from build123d import *

# Parameters (mm, degrees)
ESQUISSE1_W             = 27
ESQUISSE1_H             = 34
ESQUISSE1_R             = 10.5
BOSS_EXTRU_1_DEPTH      = 4
ESQUISSE2_W             = 27
ESQUISSE2_H             = 4
BOSS_EXTRU_2_DEPTH      = 8
BOSS_EXTRU_3_DEPTH      = 2
BOSS_EXTRU_4_DEPTH      = 2
CONG_1_R                = 10
ENL_V_MAT_EXTRU_1_DEPTH = 35.058772732


with BuildPart() as part:
    # Esquisse1 → Boss.-Extru.1 (new body)
    with BuildSketch(Plane(origin=(0, 0, 0), x_dir=(1, 0, 0), z_dir=(0, 1, 0))):
        with Locations((0.5, 3)):
            Rectangle(ESQUISSE1_W, ESQUISSE1_H)
        with Locations(Location((0, 0, 0), (0, 0, 270))):
            Circle(ESQUISSE1_R, mode=Mode.SUBTRACT)
    extrude(amount=BOSS_EXTRU_1_DEPTH)

    # Esquisse2 → Boss.-Extru.2 (add)
    with BuildSketch(Plane.XZ):
        with Locations((0.5, -18)):
            Rectangle(ESQUISSE2_W, ESQUISSE2_H)
    extrude(amount=BOSS_EXTRU_2_DEPTH)

    # Esquisse5 → Boss.-Extru.3 (add)
    with BuildSketch(Plane.ZY.offset(13)):
        Polygon((-16, 0), (-16, -5), (-11, 0), align=None)
    extrude(amount=-BOSS_EXTRU_3_DEPTH)

    # Esquisse6 → Boss.-Extru.4 (add)
    with BuildSketch(Plane(origin=(14, 0, 0), x_dir=(0, 0, -1), z_dir=(1, 0, 0))):
        Polygon((16, 0), (11, 0), (16, -5), align=None)
    extrude(amount=-BOSS_EXTRU_4_DEPTH)

    # Congé1
    cong_1_edges = [part.edges().sort_by_distance(p)[0] for p in [
        (-13, 2, 14),
        (14, 2, 14),
    ]]
    fillet(cong_1_edges, radius=CONG_1_R)

    # Esquisse7 → Enlèv. mat.-Extru.1 (cut, through all)
    with BuildSketch(Plane.XY.offset(-16)):
        with BuildLine():
            Line((-8, -2), (9, -2))
            ThreePointArc((9, -2), (11, -4), (9, -6))
            Line((9, -6), (-8, -6))
            ThreePointArc((-8, -6), (-10, -4), (-8, -2))
        make_face()
    extrude(amount=-ENL_V_MAT_EXTRU_1_DEPTH, mode=Mode.SUBTRACT)


solid = part.part
Here's how the part is built. I have some questions about the finished solid (model axes, mm). A direction names the side the tool comes from. Round coordinates to 2 decimals unless told otherwise and drop trailing zeros. Loops run counter-clockwise (first coordinate to the right, second up) from the corner with the lowest first, then second, coordinate; pieces in that order, holes last.
1. If we section it at B-B on y = -4: Write out the boundary of the cut face in (x, z).
Answer list:
outline: (-13, -20) - (-10, -20) - (-10, -16) - (-11, -16) - (-11, -15) - (-13, -15) - close; (11, -20) - (14, -20) - (14, -15) - (12, -15) - (12, -16) - (11, -16) - close
2. If we section it at A-A on z = 0: Write out the boundary of the cut face in (x, y).
Answer list:
outline: (-13, 0) - (-10.5, 0) - (-10.5, 4) - (-13, 4) - close; (10.5, 0) - (14, 0) - (14, 4) - (10.5, 4) - close
3. We'd pull the mould along Y, two halves only. Please class faces 1 (the face through (0, -2, -18)), 2 (the face through (-13, 1, -11)), 3 (the face through (0, 4, -11)): +Y half, -Y half, draft (parallel to the pull), parting line (faces both ways), or undercut.
Answer list:
face 1: undercut
face 2: draft
face 3: +Y half
4. If I drill on line 1 along Y through (x, z) = (-7, -17.5); line 2 along X through (y, z) = (2.95, 0); line 3 along X through (y, z) = (0.75, 9.5), over which ranges is the centre line in solid material (lowest first)?
Answer list:
line 1: y = -8 to -6, -2 to 4
line 2: x = -13 to -10.5, 10.5 to 14
line 3: x = -11.35 to -4.47, 4.47 to 12.35
5. Which directions (+Z, -Z, +X, -X, +Y, -Y) give clear straight access to the entire face, cutting with the end or side of a thin tool? Please do faces 4 (the face through (0, 2, 14)), 5 (the face through (0, -7, -16)), 6 (the face through (-10, -4, -18)).
Answer list:
face 4: +Z, +X, -X, +Y, -Y
face 5: +Z, -Y
face 6: +Z, -Z
6. If we section it at C-C on x = -7.25: Write out the boundary of the cut face in (y, z), plus the area to 3 significant figures.
Answer list:
outline: (-8, -20) - (-6, -20) - (-6, -16) - (-8, -16) - close; (-2, -20) - (4, -20) - (4, -7.6) - (0, -7.6) - (0, -16) - (-2, -16) - close; (0, 7.6) - (4, 7.6) - (4, 13.05) - (0, 13.05) - close
area: 87.4 mm2
7. If we section it at D-D on z = -8.5: Write out the boundary of the cut face in (x, y).
Answer list:
outline: (-13, 0) - (-6.16, 0) - (-6.16, 4) - (-13, 4) - close; (6.16, 0) - (14, 0) - (14, 4) - (6.16, 4) - close
8. For P1, Ø4, axis at x = -8, z = 0, coming from the -Y side, with a flat end and sliding along its axis, tell me the tip position at first contact or that it passes through.
Answer list:
P1: passes through
